```python
from build123d import *

# Parameters (mm, degrees)
SKETCH_W        = 80.5
SKETCH_H        = 70
PAD_DEPTH       = 3
FILLET_R        = 4.5
SKETCH001_R     = 1.75
POCKET_DEPTH    = 3.001
PAD001_DEPTH    = 5
POCKET001_DEPTH = 3.001


with BuildPart() as part:
    # Sketch → Pad (new body)
    with BuildSketch(Plane.XY):
        Rectangle(SKETCH_W, SKETCH_H)
    extrude(amount=PAD_DEPTH)

    # Fillet
    fillet_edges = [part.edges().sort_by_distance(p)[0] for p in [
        (-40.25, -35, 1.5),
        (40.25, -35, 1.5),
        (40.25, 35, 1.5),
        (-40.25, 35, 1.5),
    ]]
    fillet(fillet_edges, radius=FILLET_R)

    # Sketch001 (on Face5 of Fillet) → Pocket (cut, through all)
    with BuildSketch(Plane.XY.offset(3)):
        with Locations((-35.75, 30.5)):
            Circle(SKETCH001_R)
        with Locations((35.75, 30.5)):
            Circle(SKETCH001_R)
        with Locations((-35.75, -30.5)):
            Circle(SKETCH001_R)
        with Locations((35.75, -30.5)):
            Circle(SKETCH001_R)
    extrude(amount=-POCKET_DEPTH, mode=Mode.SUBTRACT)

    # Sketch002 (on Face5 of Pocket) → Pad001 (join)
    with BuildSketch(Plane.XY.offset(3)):
        with BuildLine():
            Line((-32.480826, -31.75), (32.480826, -31.75))
            ThreePointArc((32.395898, -29.5), (32.252491, -30.632016), (32.480826, -31.75))
            Line((-32.395898, -29.5), (32.395898, -29.5))
            ThreePointArc((-32.480826, -31.75), (-32.253104, -30.631993), (-32.395898, -29.5))
        make_face()
    pad001 = extrude(amount=PAD001_DEPTH)

    # Mirrored: Pad001 across XZ
    add(pad001.mirror(Plane.XZ))

    # Sketch003 (on Face5 of Mirrored) → Pocket001 (cut, through all)
    with BuildSketch(Plane.XY.offset(3)):
        Polygon((34.75, 25.5), (34.75, -25.5), (-28.75, -25.5), (-28.75, -13.75), (-31.25, -11.25), (-31.25, 21.75), (-28.75, 24.25), (-28.75, 25.5), align=None)
    extrude(amount=-POCKET001_DEPTH, mode=Mode.SUBTRACT)


solid = part.part
```
For this review, take the finished solid that the model builds, in its own axes (mm). A direction names the side the tool comes from. Round coordinates to 2 decimals unless told otherwise and drop trailing zeros. Write each loop counter-clockwise with the first axis right and the second up, starting at its lowest first coordinate (ties: lowest second). Pieces come first, ordered by that corner, then holes. Notation, with made-up numbers: M 79.25,-30.5 L 112.25,-30.5 A34 ccw 112.25,3.5 Z; hole C 77,45.5 d4. An arc over 180 degrees is marked long. One line per item, written item: value. Start each with the question number.
(1) The part is to be moulded in two halves that separate along X. For faces 5 (the cylindrical face through (-38.967, -33.647, 1.521)), 6 (the flat face through (0, 31.75, 5)), 7 (the cylindrical face through (-34.133, -31.17, 1.521)), 8 (the flat face through (-28.75, -20, 2)), say which applies: released by +X, released by -X, zero draft, split by the parting line, or undercut.
(2) We need section B-B (x = -15). Give the boundary of the cut face in (y, z).
(3) Wall thickness on line 1 (Y direction, x = 35.75, z = 1.05); line 2 (Y direction, x = 17.5, z = 2.5); line 3 (Y direction, x = 21, z = 7.75): over which ranges is each line inside the solid? List them lowest first.
(4) Insertion check: pin 1 (2.5 mm diameter, centred on x = 2, z = 6.5, fed in from -Y); pin 2 (1 mm diameter, centred on x = 12, z = 6.5, fed in from +Y); pin 3 (5.5 mm diameter, centred on x = 35.75, y = -30.5, fed in from +Z). Each pin has a flat end and moves straight along its axis. Give the tip position at first contact, or say it passes through.
(5) We need section A-A (y = -9.5). Give the boundary of the cut face in (x, z), and give its area (3 significant figures).
(6) We need section C-C (y = 27.5). Give the boundary of the cut face in (x, z), and give its area (4 significant figures).
(7) Machinability: for faces 1 (the flat face through (34.75, 0, 2)), 2 (the flat face through (0, -31.75, 5)), 3 (the cylindrical face through (32.252, 30.616, 5.465)), 4 (the flat face through (0, -29.5, 5)), which of the approach directions +Z, -Z, +X, -X, +Y, -Y give a long, thin tool a straight path to every point of the face, cutting with its end or side? Answer none if there is none.
Result:
1. face 5: released by -X
1. face 6: zero draft
1. face 7: undercut
1. face 8: undercut
2. outline: M -35,0 L -25.5,0 L -25.5,3 L -29.5,3 L -29.5,8 L -31.75,8 L -31.75,3 L -35,3 Z; M 25.5,0 L 35,0 L 35,3 L 31.75,3 L 31.75,8 L 29.5,8 L 29.5,3 L 25.5,3 Z
3. line 1: -35 to -32.25, -28.75 to 28.75, 32.25 to 35
3. line 2: -35 to -25.5, 25.5 to 35
3. line 3: -31.75 to -29.5, 29.5 to 31.75
4. pin 1: y = -31.75
4. pin 2: y = 31.75
4. pin 3: z = 3
5. outline: M -40.25,0 L -31.25,0 L -31.25,3 L -40.25,3 Z; M 34.75,0 L 40.25,0 L 40.25,3 L 34.75,3 Z
5. area: 43.5 mm²
6. outline: M -40.25,0 L 40.25,0 L 40.25,3 L -40.25,3 Z
6. area: 241.5 mm²
7. face 1: +Z, -Z
7. face 2: +Z, +X, -X, -Y
7. face 3: +Z, +X
7. face 4: +Z, +X, -X
